```python
from build123d import *

# Parameters (mm, degrees)
F1_DEPTH = 6


with BuildPart() as f1:
    # F0 (on Front) → F1 (new body)
    with BuildSketch(Plane.XZ):
        Polygon((-65.540905, -63.527275), (-67.540905, -61.527275), (-101.540905, -61.527275), (-103.540905, -63.527275), (-103.540905, -128.527275), (-101.540905, -130.527275), (-67.540905, -130.527275), (-65.540905, -128.527275), align=None)
        with BuildLine():
            ThreePointArc((-95.540905, -121.327275), (-97.874357, -120.360727), (-98.840905, -118.027275))
            ThreePointArc((-98.840905, -118.027275), (-97.874357, -115.693823), (-95.540905, -114.727275))
            ThreePointArc((-95.540905, -114.727275), (-93.207453, -115.693823), (-92.240905, -118.027275))
            ThreePointArc((-92.240905, -118.027275), (-93.207453, -120.360727), (-95.540905, -121.327275))
        make_face(mode=Mode.SUBTRACT)
        with BuildLine():
            ThreePointArc((-73.540905, -121.327275), (-75.874357, -120.360727), (-76.840905, -118.027275))
            ThreePointArc((-76.840905, -118.027275), (-75.874357, -115.693823), (-73.540905, -114.727275))
            ThreePointArc((-73.540905, -114.727275), (-71.207453, -115.693823), (-70.240905, -118.027275))
            ThreePointArc((-70.240905, -118.027275), (-71.207453, -120.360727), (-73.540905, -121.327275))
        make_face(mode=Mode.SUBTRACT)
        with BuildLine():
            ThreePointArc((-84.540905, -74.327275), (-86.874357, -73.360727), (-87.840905, -71.027275))
            ThreePointArc((-87.840905, -71.027275), (-86.874357, -68.693823), (-84.540905, -67.727275))
            ThreePointArc((-84.540905, -67.727275), (-82.207453, -68.693823), (-81.240905, -71.027275))
            ThreePointArc((-81.240905, -71.027275), (-82.207453, -73.360727), (-84.540905, -74.327275))
        make_face(mode=Mode.SUBTRACT)
    extrude(amount=-F1_DEPTH)


solid = f1.part
```
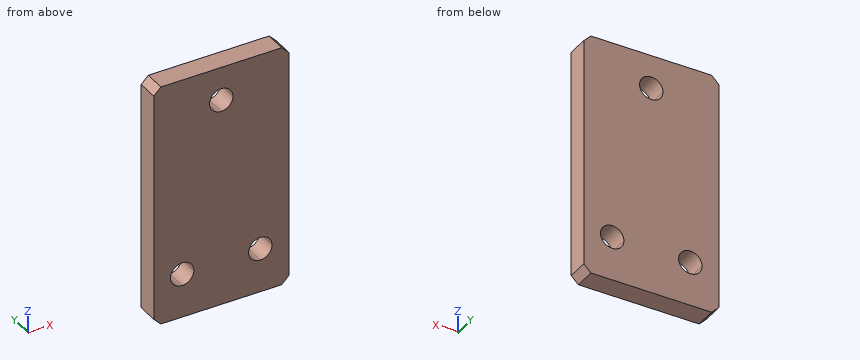
Work out the finished part from the listing and answer in its coordinate system (mm). Round coordinates to 2 decimals unless told otherwise and drop trailing zeros. Loops run counter-clockwise (first coordinate to the right, second up) from the corner with the lowest first, then second, coordinate; pieces in that order, holes last. Notation, with made-up numbers: (43.25, -17.5) -> (75.25, -17.5) arc R24 ccw to (75.25, 12.5) -> close; hole circle Ø4 at (5.5, 63.5). An arc over 180 degrees is marked (long way). Write each question's results on one line, items separated by ' | '. Start each with the question number.
1. Section A-A (y = 1.7) is taken. Determine the outline of the cut face in (x, z).
2. Section B-B (x = -72.5) is taken. Determine the outline of the cut face in (y, z), plus the area to 3 significant figures.
3. Section C-C (z = -116) is taken. Determine the outline of the cut face in (x, y).
4. Find the intervals of material crossed by probe 1 along Z at (x, y) = (-95.5, 3.6); probe 2 along Z at (x, y) = (-96, 3.5); probe 3 along X at (y, z) = (2.1, -120.5), in increasing order. Write a range as from..to.
5. Given pin 1 Ø5 at (x, z) = (-95, -84) entering from -Y, flat-ended and moving along its own axis, determine where the tip first touches the part or whether it passes through.
Evaluation:
1) outline: (-103.54, -128.53) -> (-101.54, -130.53) -> (-67.54, -130.53) -> (-65.54, -128.53) -> (-65.54, -63.53) -> (-67.54, -61.53) -> (-101.54, -61.53) -> (-103.54, -63.53) -> close; hole (-98.84, -118.03) arc R3.3 ccw to (-95.54, -121.33) arc R3.3 ccw to (-92.24, -118.03) arc R3.3 ccw to (-95.54, -114.73) arc R3.3 ccw to start; hole (-87.84, -71.03) arc R3.3 ccw to (-84.54, -74.33) arc R3.3 ccw to (-81.24, -71.03) arc R3.3 ccw to (-84.54, -67.73) arc R3.3 ccw to start; hole (-76.84, -118.03) arc R3.3 ccw to (-73.54, -121.33) arc R3.3 ccw to (-70.24, -118.03) arc R3.3 ccw to (-73.54, -114.73) arc R3.3 ccw to start
2) outline: (0, -130.53) -> (6, -130.53) -> (6, -121.16) -> (0, -121.16) -> close; (0, -114.9) -> (6, -114.9) -> (6, -61.53) -> (0, -61.53) -> close | area: 376 mm2
3) outline: (-103.54, 0) -> (-98.14, 0) -> (-98.14, 6) -> (-103.54, 6) -> close; (-92.94, 0) -> (-76.14, 0) -> (-76.14, 6) -> (-92.94, 6) -> close; (-70.94, 0) -> (-65.54, 0) -> (-65.54, 6) -> (-70.94, 6) -> close
4) probe 1: z = -130.53..-121.33, -114.73..-61.53 | probe 2: z = -130.53..-121.3, -114.76..-61.53 | probe 3: x = -103.54..-97.73, -93.36..-75.73, -71.36..-65.54
5) pin 1: stops at y = 0
